Geometry: final body of the model. Coordinates: model frame, mm. Round coordinates to 2 decimals unless told otherwise and drop trailing zeros. Loops run counter-clockwise (first coordinate to the right, second up) from the corner with the lowest first, then second, coordinate; pieces in that order, holes last. Notation, with made-up numbers: M -11,-20.75 L 17,-20.75 A20 ccw 17,-8.75 Z; hole C 66,83 d2. An arc over 180 degrees is marked long. Answer as a JSON object with one key per item and string values.
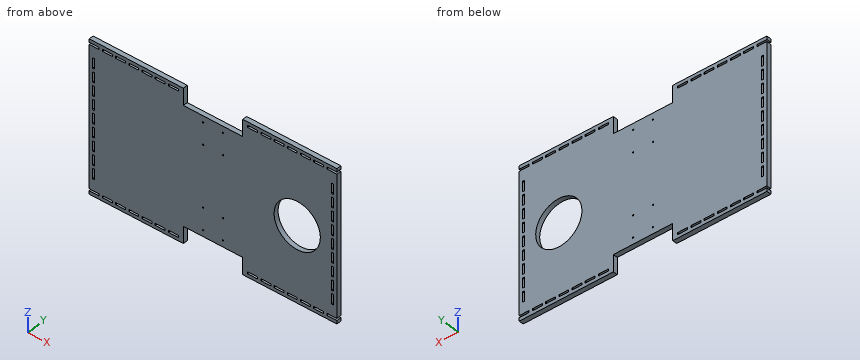
from build123d import *

# Parameters (mm, degrees)
SKETCH6_W           = 15
SKETCH6_H           = 3
SKETCH6_W_2         = 3
SKETCH6_H_2         = 15
SKETCH6_R           = 1
SKETCH6_R_2         = 35
BOSS_EXTRUDE3_DEPTH = 7


with BuildPart() as part:
    # Sketch6 → Boss-Extrude3 (new body)
    with BuildSketch(Plane(origin=(0, 0, 0), x_dir=(1, 0, 0), z_dir=(0, 1, 0))):
        Polygon((-45, 112.5), (-187.5, 112.5), (-187.5, 107.5), (-172.5, 107.5), (-172.5, 104.5), (-187.5, 104.5), (-187.5, -104.5), (-172.5, -104.5), (-172.5, -107.5), (-187.5, -107.5), (-187.5, -112.5), (-45, -112.5), (-45, -87.5), (45, -87.5), (45, -112.5), (187.5, -112.5), (187.5, -107.5), (172.5, -107.5), (172.5, -104.5), (187.5, -104.5), (187.5, 104.5), (172.5, 104.5), (172.5, 107.5), (187.5, 107.5), (187.5, 112.5), (45, 112.5), (45, 87.5), (-45, 87.5), align=None)
        with Locations((-160, -106)):
            Rectangle(SKETCH6_W, SKETCH6_H, mode=Mode.SUBTRACT)
        with Locations((-140, -106)):
            Rectangle(SKETCH6_W, SKETCH6_H, mode=Mode.SUBTRACT)
        with Locations((-120, -106)):
            Rectangle(SKETCH6_W, SKETCH6_H, mode=Mode.SUBTRACT)
        with Locations((-100, -106)):
            Rectangle(SKETCH6_W, SKETCH6_H, mode=Mode.SUBTRACT)
        with Locations((-181, -80)):
            Rectangle(SKETCH6_W_2, SKETCH6_H_2, mode=Mode.SUBTRACT)
        with Locations((-181, -60)):
            Rectangle(SKETCH6_W_2, SKETCH6_H_2, mode=Mode.SUBTRACT)
        with Locations((-80, -106)):
            Rectangle(SKETCH6_W, SKETCH6_H, mode=Mode.SUBTRACT)
        with Locations((-60, -106)):
            Rectangle(SKETCH6_W, SKETCH6_H, mode=Mode.SUBTRACT)
        with Locations(Location((-15, -77.920021532, 0), (0, 0, 270))):
            Circle(SKETCH6_R, mode=Mode.SUBTRACT)
        with Locations((-181, -40)):
            Rectangle(SKETCH6_W_2, SKETCH6_H_2, mode=Mode.SUBTRACT)
        with Locations((-181, -20)):
            Rectangle(SKETCH6_W_2, SKETCH6_H_2, mode=Mode.SUBTRACT)
        with Locations(Location((-15, -45.520021532, 0), (0, 0, 270))):
            Circle(SKETCH6_R, mode=Mode.SUBTRACT)
        with Locations((60, -106)):
            Rectangle(SKETCH6_W, SKETCH6_H, mode=Mode.SUBTRACT)
        with Locations((80, -106)):
            Rectangle(SKETCH6_W, SKETCH6_H, mode=Mode.SUBTRACT)
        with Locations(Location((15, -77.920021532, 0), (0, 0, 270))):
            Circle(SKETCH6_R, mode=Mode.SUBTRACT)
        with Locations((100, -106)):
            Rectangle(SKETCH6_W, SKETCH6_H, mode=Mode.SUBTRACT)
        with Locations((120, -106)):
            Rectangle(SKETCH6_W, SKETCH6_H, mode=Mode.SUBTRACT)
        with Locations((140, -106)):
            Rectangle(SKETCH6_W, SKETCH6_H, mode=Mode.SUBTRACT)
        with Locations((160, -106)):
            Rectangle(SKETCH6_W, SKETCH6_H, mode=Mode.SUBTRACT)
        with Locations((181, -80)):
            Rectangle(SKETCH6_W_2, SKETCH6_H_2, mode=Mode.SUBTRACT)
        with Locations((181, -60)):
            Rectangle(SKETCH6_W_2, SKETCH6_H_2, mode=Mode.SUBTRACT)
        with Locations(Location((15, -45.520021532, 0), (0, 0, 270))):
            Circle(SKETCH6_R, mode=Mode.SUBTRACT)
        with Locations((181, -40)):
            Rectangle(SKETCH6_W_2, SKETCH6_H_2, mode=Mode.SUBTRACT)
        with Locations((181, -20)):
            Rectangle(SKETCH6_W_2, SKETCH6_H_2, mode=Mode.SUBTRACT)
        with Locations((-181, 0)):
            Rectangle(SKETCH6_W_2, SKETCH6_H_2, mode=Mode.SUBTRACT)
        with Locations((-181, 20)):
            Rectangle(SKETCH6_W_2, SKETCH6_H_2, mode=Mode.SUBTRACT)
        with Locations((-181, 40)):
            Rectangle(SKETCH6_W_2, SKETCH6_H_2, mode=Mode.SUBTRACT)
        with Locations(Location((-15, 45.520021532, 0), (0, 0, 270))):
            Circle(SKETCH6_R, mode=Mode.SUBTRACT)
        with Locations((-181, 60)):
            Rectangle(SKETCH6_W_2, SKETCH6_H_2, mode=Mode.SUBTRACT)
        with Locations((-181, 80)):
            Rectangle(SKETCH6_W_2, SKETCH6_H_2, mode=Mode.SUBTRACT)
        with Locations((-160, 106)):
            Rectangle(SKETCH6_W, SKETCH6_H, mode=Mode.SUBTRACT)
        with Locations((-140, 106)):
            Rectangle(SKETCH6_W, SKETCH6_H, mode=Mode.SUBTRACT)
        with Locations((-120, 106)):
            Rectangle(SKETCH6_W, SKETCH6_H, mode=Mode.SUBTRACT)
        with Locations((-100, 106)):
            Rectangle(SKETCH6_W, SKETCH6_H, mode=Mode.SUBTRACT)
        with Locations(Location((-15, 77.920021532, 0), (0, 0, 270))):
            Circle(SKETCH6_R, mode=Mode.SUBTRACT)
        with Locations((-80, 106)):
            Rectangle(SKETCH6_W, SKETCH6_H, mode=Mode.SUBTRACT)
        with Locations((-60, 106)):
            Rectangle(SKETCH6_W, SKETCH6_H, mode=Mode.SUBTRACT)
        with Locations(Location((15, 45.520021532, 0), (0, 0, 270))):
            Circle(SKETCH6_R, mode=Mode.SUBTRACT)
        with Locations(Location((127.5, 0, 0), (0, 0, 270))):
            Circle(SKETCH6_R_2, mode=Mode.SUBTRACT)
        with Locations((181, 0)):
            Rectangle(SKETCH6_W_2, SKETCH6_H_2, mode=Mode.SUBTRACT)
        with Locations((181, 20)):
            Rectangle(SKETCH6_W_2, SKETCH6_H_2, mode=Mode.SUBTRACT)
        with Locations((181, 40)):
            Rectangle(SKETCH6_W_2, SKETCH6_H_2, mode=Mode.SUBTRACT)
        with Locations(Location((15, 77.920021532, 0), (0, 0, 270))):
            Circle(SKETCH6_R, mode=Mode.SUBTRACT)
        with Locations((60, 106)):
            Rectangle(SKETCH6_W, SKETCH6_H, mode=Mode.SUBTRACT)
        with Locations((80, 106)):
            Rectangle(SKETCH6_W, SKETCH6_H, mode=Mode.SUBTRACT)
        with Locations((181, 60)):
            Rectangle(SKETCH6_W_2, SKETCH6_H_2, mode=Mode.SUBTRACT)
        with Locations((181, 80)):
            Rectangle(SKETCH6_W_2, SKETCH6_H_2, mode=Mode.SUBTRACT)
        with Locations((100, 106)):
            Rectangle(SKETCH6_W, SKETCH6_H, mode=Mode.SUBTRACT)
        with Locations((120, 106)):
            Rectangle(SKETCH6_W, SKETCH6_H, mode=Mode.SUBTRACT)
        with Locations((140, 106)):
            Rectangle(SKETCH6_W, SKETCH6_H, mode=Mode.SUBTRACT)
        with Locations((160, 106)):
            Rectangle(SKETCH6_W, SKETCH6_H, mode=Mode.SUBTRACT)
    extrude(amount=BOSS_EXTRUDE3_DEPTH)


solid = part.part
1) Pin query (flat end, axial travel): P1, Ø0.9, axis at y = 3.5, z = -106.5, coming from the -X side. Return the tip coordinate at first contact, or that it passes through.
Results:
{"P1": "x = -172.5"}
2) Section query A-A (z = -63). Return the cut outline in (x, y), and give its area (3 significant figures).
Results:
{"outline": "M -187.5,0 L -182.5,0 L -182.5,7 L -187.5,7 Z; M -179.5,0 L 179.5,0 L 179.5,7 L -179.5,7 Z; M 182.5,0 L 187.5,0 L 187.5,7 L 182.5,7 Z", "area": "2,580 mm2"}
3) Section query B-B (x = -61). Return the cut outline in (y, z).
Results:
{"outline": "M 0,-112.5 L 7,-112.5 L 7,-107.5 L 0,-107.5 Z; M 0,-104.5 L 7,-104.5 L 7,104.5 L 0,104.5 Z; M 0,107.5 L 7,107.5 L 7,112.5 L 0,112.5 Z"}
4) Section query D-D (x = 116). Return the cut outline in (y, z).
Results:
{"outline": "M 0,-112.5 L 7,-112.5 L 7,-107.5 L 0,-107.5 Z; M 0,-104.5 L 7,-104.5 L 7,-33.06 L 0,-33.06 Z; M 0,33.06 L 7,33.06 L 7,104.5 L 0,104.5 Z; M 0,107.5 L 7,107.5 L 7,112.5 L 0,112.5 Z"}
5) Section query C-C (z = 93.5). Return the cut outline in (x, y), and give its area (4 significant figures).
Results:
{"outline": "M -187.5,0 L -45,0 L -45,7 L -187.5,7 Z; M 45,0 L 187.5,0 L 187.5,7 L 45,7 Z", "area": "1,995 mm2"}
6) Ray query, line 1 (X direction, y = 6.5, z = -53); line 2 (X direction, y = 2.5, z = -92); line 3 (Z direction, x = -64, y = 4.25). Return the intervals inside material, ascending.
Results:
{"line 1": "-187.5 to -182.5, -179.5 to 179.5, 182.5 to 187.5", "line 2": "-187.5 to -45, 45 to 187.5", "line 3": "-112.5 to -107.5, -104.5 to 104.5, 107.5 to 112.5"}
